```python
from build123d import *

# Parameters (mm, degrees)
SKETCH1_R           = 3.130555183
BOSS_EXTRUDE1_DEPTH = 5
SKETCH2_R           = 1.6
CUT_EXTRUDE1_DEPTH  = 10


with BuildPart() as part:
    # Sketch1 → Boss-Extrude1 (new body)
    with BuildSketch(Plane.XY):
        with BuildLine():
            Line((7, 270), (7, 0))
            ThreePointArc((7, 0), (0, -7), (-7, 0))
            Line((-7, 0), (-7, 270))
            ThreePointArc((-7, 270), (0, 277), (7, 270))
        make_face()
        Circle(SKETCH1_R, mode=Mode.SUBTRACT)
    extrude(amount=BOSS_EXTRUDE1_DEPTH)

    # Sketch2 → Cut-Extrude1 (cut)
    with BuildSketch(Plane.XY.offset(5)):
        with Locations((0, 270)):
            Circle(SKETCH2_R)
        with Locations((0, 260)):
            Circle(SKETCH2_R)
    extrude(amount=-CUT_EXTRUDE1_DEPTH, mode=Mode.SUBTRACT)


solid = part.part
```
Design review of the part built by this model. Coordinates are the model's own, in mm. Coordinates: 2 decimals unless noted, no trailing zeros. Write each loop counter-clockwise with the first axis right and the second up, starting at its lowest first coordinate (ties: lowest second). Pieces come first, ordered by that corner, then holes. Notation, with made-up numbers: M 4.5,40 L 24.5,40 A27 cw 24.5,60 Z; hole C 87,23 d5. An arc over 180 degrees is marked long. Answer as a JSON object with one key per item and string values.
Item 1: Add section A-A, the plane z = 1.3. Give the boundary of the cut face in (x, y), and give its area (3 significant figures).
Outcome:
{"outline": "M -7,0 A7 ccw 7,0 L 7,270 A7 ccw -7,270 Z; hole C 0,0 d6.26; hole C 0,260 d3.2; hole C 0,270 d3.2", "area": "3,890 mm²"}
Item 2: Insertion check: pin 1 Ø2 at (x, z) = (5, 2.5) entering from +Y; pin 2 Ø5 at (x, y) = (-4, 162) entering from -Z. Each pin has a flat end and moves straight along its axis. Give the tip position at first contact, or say it passes through.
Outcome:
{"pin 1": "y = 275.74", "pin 2": "z = 0"}
Item 3: Wall thickness on probe 1 along Y at (x, z) = (0, 3.15); probe 2 along X at (y, z) = (270, 3.05); probe 3 along Y at (x, z) = (0.75, 1.4): over which ranges is each line inside the solid? List them lowest first.
Outcome:
{"probe 1": "-7 to -3.13, 3.13 to 258.4, 261.6 to 268.4, 271.6 to 277", "probe 2": "-7 to -1.6, 1.6 to 7", "probe 3": "-6.96 to -3.04, 3.04 to 258.59, 261.41 to 268.59, 271.41 to 276.96"}
Item 4: Draft analysis for pull direction X (two halves, no side actions). For faces 1 (the cylindrical face through (-0.679, -3.056, 2.465)), 2 (the cylindrical face through (0, 277, 2)), 3 (the flat face through (7, 137, 2)), state which applies: pulls with the +X half, pulls with the -X half, needs draft (parallel to the pull), parting line crosses it, or undercut.
Outcome:
{"face 1": "undercut", "face 2": "parting line crosses it", "face 3": "pulls with the +X half"}
